Check sheet for the modelled part. Datum: model origin and axes. Units: mm. A direction names the side the tool comes from. Give positions to 0.01 mm unless a question says otherwise; leave off trailing zeros. Write each loop counter-clockwise with the first axis right and the second up, starting at its lowest first coordinate (ties: lowest second). Pieces come first, ordered by that corner, then holes. Notation, with made-up numbers: (20.5, 61) -> (52.5, 61) arc R7 cw to (52.5, 68) -> close; hole circle Ø7 at (77.5, 14). An arc over 180 degrees is marked (long way). Answer as a JSON object with one key per item and string values.
from build123d import *

# Parameters (mm, degrees)
BOSS_EXTRUDE1_DEPTH     = 10
CUT_EXTRUDE1_REACH      = 68.078
SKETCH2_R               = 5
CUT_EXTRUDE2_REACH      = 69.457
CUT_EXTRUDE2_END_RADIUS = 31.503056099
SKETCH3_R               = 5


with BuildPart() as part:
    # Sketch1 → Boss-Extrude1 (new, symmetric)
    with BuildSketch(Plane(origin=(0, 0, 0), x_dir=(1, 0, 0), z_dir=(0, 1, 0))):
        with BuildLine():
            Line((29, 10.842426248), (29, -10.842426248))
            ThreePointArc((29, -10.842426248), (0, -30.039282951), (-29, -10.842426248))
            Line((-29, -10.842426248), (-29, 10.842426248))
            ThreePointArc((-29, 10.842426248), (0, 30.039282951), (29, 10.842426248))
        make_face()
        with BuildLine():
            Line((-25, 10), (-25, -10))
            ThreePointArc((-25, -10), (0, -26.039282951), (25, -10))
            Line((25, -10), (25, 10))
            ThreePointArc((25, 10), (0, 26.039282951), (-25, 10))
        make_face(mode=Mode.SUBTRACT)
    extrude(amount=BOSS_EXTRUDE1_DEPTH, both=True)

    # Cut-Extrude1: up to this face of the body (flat: up to its plane)
    cut_extrude1_end = Plane(part.part.faces().sort_by_distance((29, 0, 0))[0])
    # Sketch2 → Cut-Extrude1 (cut, up to the picked face)
    with BuildSketch(Plane.ZY.offset(29), mode=Mode.PRIVATE) as cut_extrude1_sk1:
        Circle(SKETCH2_R)
    cut_extrude1_tool1 = split(extrude(cut_extrude1_sk1.sketch, amount=-CUT_EXTRUDE1_REACH, mode=Mode.PRIVATE), bisect_by=cut_extrude1_end, keep=Keep.BOTH, mode=Mode.PRIVATE)
    add(cut_extrude1_tool1.solids().sort_by(Axis((-29, 0, 0), (1, 0, 0)))[0], mode=Mode.SUBTRACT)

    # Cut-Extrude2: up to this cylinder (the profile starts inside it)
    cut_extrude2_end = Plane(origin=(0, 2.5, 1.463773147), z_dir=(0, -1, 0)) * Cylinder(CUT_EXTRUDE2_END_RADIUS, 202.920112198, mode=Mode.PRIVATE)
    # Sketch3 → Cut-Extrude2 (cut, up to the surface)
    with BuildSketch(Plane.XY.offset(30.039282951), mode=Mode.PRIVATE) as cut_extrude2_sk1:
        with Locations((0, 2.5)):
            Circle(SKETCH3_R)
    cut_extrude2_tool1 = extrude(cut_extrude2_sk1.sketch, amount=-CUT_EXTRUDE2_REACH, mode=Mode.PRIVATE) & cut_extrude2_end
    add(cut_extrude2_tool1.solids().sort_by_distance((0, 2.5, 30.039283))[0], mode=Mode.SUBTRACT)


solid = part.part
1. Sectioned sample at C-C, the plane z = 0. Enter the section's corners in (x, y).
Determined:
{"outline": "(-29, -10) -> (-25, -10) -> (-25, -5) -> (-29, -5) -> close; (-29, 5) -> (-25, 5) -> (-25, 10) -> (-29, 10) -> close; (25, -10) -> (29, -10) -> (29, -5) -> (25, -5) -> close; (25, 5) -> (29, 5) -> (29, 10) -> (25, 10) -> close"}
2. Sectioned sample at D-D, the plane x = 0. Enter the section's corners in (y, z), plus the area to 3 significant figures.
Determined:
{"outline": "(-10, -30.04) -> (-2.5, -30.04) -> (-2.5, -26.04) -> (-10, -26.04) -> close; (-10, 26.04) -> (-2.5, 26.04) -> (-2.5, 30.04) -> (-10, 30.04) -> close; (7.5, -30.04) -> (10, -30.04) -> (10, -26.04) -> (7.5, -26.04) -> close; (7.5, 26.04) -> (10, 26.04) -> (10, 30.04) -> (7.5, 30.04) -> close", "area": "80.0 mm^2"}
3. Scan lines: L1, parallel to X at y = 5.25, z = -5; L2, parallel to Y at x = 27.75, z = 0; L3, parallel to Y at x = 0, z = -27.7. Record each from-to range of solid material in increasing order. Write a range as [from, to].
Determined:
{"L1": "[-29, -25], [25, 29]", "L2": "[-10, -5], [5, 10]", "L3": "[-10, -2.5], [7.5, 10]"}
4. Mould release check, pull along Y, two halves, no side actions. Record for faces 1 (the face through (-27.03, -4.88, -1.08)), 2 (the face through (29, 5, -3)), 3 (the face through (-0.651, 7.457, 27.842)), 4 (the face through (26, -10, 0)): released by +Y, released by -Y, zero draft, split by the parting line, or undercut.
Determined:
{"face 1": "undercut", "face 2": "zero draft", "face 3": "undercut", "face 4": "released by -Y"}
5. Sectioned sample at A-A, the plane z = 7. Enter the section's corners in (x, y).
Determined:
{"outline": "(-29, -10) -> (-25, -10) -> (-25, 10) -> (-29, 10) -> close; (25, -10) -> (29, -10) -> (29, 10) -> (25, 10) -> close"}
6. Go/stop test with flat-tipped pins: P1, Ø5, axis at y = 2, z = 17, coming from the -X side; P2, Ø5, axis at x = 21.5, y = -6.5, coming from the +Z side; P3, Ø6, axis at y = -8, z = 23, coming from the -X side. Record where each tip stops, or that it passes through.
Determined:
{"P1": "x = -27.16", "P2": "z = 23.66", "P3": "x = -23.06"}
7. Sectioned sample at B-B, the plane y = 8.25. Enter the section's corners in (x, z), plus the area to 4 significant figures.
Determined:
{"outline": "(-29, -10.84) arc R31.5 ccw to (29, -10.84) -> (29, 10.84) arc R31.5 ccw to (-29, 10.84) -> close; hole (-25, -10) arc R27.5 ccw to (25, -10) -> (25, 10) arc R27.5 ccw to (-25, 10) -> close", "area": "712.5 mm^2"}
8. Access from +Z, -Z, +X, -X, +Y, -Y to the whole of each face (thin tool, end or side, straight path). Record for faces 5 (the face through (0.439, -4.304, -26.036)), 6 (the face through (-0.516, -4.304, -30.035)).
Determined:
{"face 5": "+Y, -Y", "face 6": "-Z, +Y, -Y"}
